from build123d import *

# Parameters (mm, degrees)
EXTRUDE_1_DEPTH          = 2.3
EXTRUDE_1_DEPTH_BACK     = 2.3
EXTRUDE_2_DEPTH          = 1.4
EXTRUDE_3_DEPTH          = 2
EXTRUDE_3_DEPTH_BACK     = 2
CUT_EXTRUDE_2_DEPTH      = 7.4
CUT_EXTRUDE_3_DEPTH      = 2
CUT_EXTRUDE_3_DEPTH_BACK = 2
FILLET_1_R               = 0.2
FILLET_2_R               = 0.1


with BuildPart() as part:
    # 草图1 → 凸台-拉伸1 (new, two sides: drawn at the far end of the back side and taken through both)
    with BuildSketch(Plane.XY.offset(-EXTRUDE_1_DEPTH_BACK)):
        Polygon((0, 0), (-14.8, 0), (-14.8, 1.3), (0, 1.3), (5.65072033, 1.3), (2.420449835, 19.619774331), (-0.822713256, 23.484825595), (-1.2165133, 23.484825595), (-1.2165133, 24.784825595), (-0.2165133, 24.784825595), (3.640212358, 20.188558937), (7.2, 0), align=None)
    extrude(amount=EXTRUDE_1_DEPTH + EXTRUDE_1_DEPTH_BACK)

    # 草图2 → 凸台-拉伸2 (add)
    with BuildSketch(Plane.XY.offset(2.3)):
        with BuildLine():
            Line((-14.8, 0), (7.2, 0))
            Line((7.2, 0), (3.640212358, 20.188558937))
            Line((3.640212358, 20.188558937), (-0.2165133, 24.784825595))
            Line((-0.2165133, 24.784825595), (-1.2165133, 24.784825595))
            ThreePointArc((-1.2165133, 24.784825595), (-2.266370135, 9.969308294), (-14.8, 2))
            Line((-14.8, 2), (-14.8, 0))
        make_face()
    extrude_2 = extrude(amount=EXTRUDE_2_DEPTH)

    # 镜向1: 凸台-拉伸2 across plane
    add(extrude_2.mirror(Plane.XY))

    # 草图4 → 凸台-拉伸3 (add, two sides: drawn at the far end of the back side and taken through both)
    with BuildSketch(Plane.XY.offset(-EXTRUDE_3_DEPTH_BACK)):
        with BuildLine():
            Line((-1.5, 0), (1.5, 0))
            Line((1.5, 0), (1.5, -0.677124344))
            ThreePointArc((1.5, -0.677124344), (1.780042303, -1.088161527), (1.95, -1.555590279))
            Line((1.95, -1.555590279), (1.95, -2.5))
            Line((1.95, -2.5), (-1.95, -2.5))
            Line((-1.95, -2.5), (-1.95, -1.555590279))
            ThreePointArc((-1.95, -1.555590279), (-1.780042303, -1.088161527), (-1.5, -0.677124344))
            Line((-1.5, -0.677124344), (-1.5, 0))
        make_face()
    extrude(amount=EXTRUDE_3_DEPTH + EXTRUDE_3_DEPTH_BACK)

    # 草图5 → 切除-拉伸2 (cut)
    with BuildSketch(Plane.XY.offset(3.7)):
        with BuildLine():
            Line((-1.2165133, 24.784825595), (-14.8, 2))
            ThreePointArc((-14.8, 2), (-2.266370135, 9.969308294), (-1.2165133, 24.784825595))
        make_face()
    extrude(amount=-CUT_EXTRUDE_2_DEPTH, mode=Mode.SUBTRACT)

    # 草图6 → 切除-拉伸3 (cut, two sides: drawn at the far end of the back side and taken through both)
    with BuildSketch(Plane(origin=(0, 0, 0), x_dir=(0, 0, -1), z_dir=(1, 0, 0)).offset(-CUT_EXTRUDE_3_DEPTH_BACK)):
        with BuildLine():
            Line((1.5, 0), (1.5, -0.677124344))
            ThreePointArc((1.5, -0.677124344), (1.780042303, -1.088161527), (1.95, -1.555590279))
            Line((1.95, -1.555590279), (1.95, -2.5))
            Line((1.95, -2.5), (2, -2.5))
            Line((2, -2.5), (2, 0))
            Line((2, 0), (1.5, 0))
        make_face()
        with BuildLine():
            Line((-1.95, -2.5), (-2, -2.5))
            Line((-2, -2.5), (-2, 0))
            Line((-2, 0), (-1.5, 0))
            Line((-1.5, 0), (-1.5, -0.677124344))
            ThreePointArc((-1.5, -0.677124344), (-1.780042303, -1.088161527), (-1.95, -1.555590279))
            Line((-1.95, -1.555590279), (-1.95, -2.5))
        make_face()
    extrude(amount=CUT_EXTRUDE_3_DEPTH + CUT_EXTRUDE_3_DEPTH_BACK, mode=Mode.SUBTRACT)

    # 圆角1
    fillet_1_edges = [part.edges().sort_by_distance(p)[0] for p in [
        (-14.8, 2, -3),
        (-14.8, 2, 3),
        (-14.8, 1, 3.7),
        (-14.8, 1, -3.7),
        (-0.7165133, 24.784825595, -3.7),
        (-0.7165133, 24.784825595, 3.7),
        (-0.2165133, 24.784825595, 0),
        (1.711849529, 22.486692266, -3.7),
        (1.711849529, 22.486692266, 3.7),
        (3.640212358, 20.188558937, 0),
        (5.420106179, 10.094279468, -3.7),
        (5.420106179, 10.094279468, 3.7),
        (7.2, 0, 0),
        (-3.8, 0, -3.7),
        (-3.8, 0, 3.7),
        (-14.8, 0, 0),
    ]]
    fillet(fillet_1_edges, radius=FILLET_1_R)

    # 圆角2
    fillet_2_edges = [part.edges().sort_by_distance(p)[0] for p in [
        (1.95, -2.5, 0),
        (-1.95, -2.5, 0),
        (0, -2.5, -1.95),
        (0, -2.5, 1.95),
    ]]
    fillet(fillet_2_edges, radius=FILLET_2_R)


solid = part.part
Input: part model. Units: mm. Frame: model coordinates. A direction names the side the tool comes from. Coordinates: 2 decimals unless noted, no trailing zeros. Write each loop counter-clockwise with the first axis right and the second up, starting at its lowest first coordinate (ties: lowest second). Pieces come first, ordered by that corner, then holes. Notation, with made-up numbers: M 34,42.5 L 84,42.5 A24 ccw 84,57.5 Z; hole C 6.25,9.5 d4. An arc over 180 degrees is marked long. Answer as a JSON object with one key per item and string values. Group by question number.
(1) Section B-B on x = -2.5. Output: boundary loops of the cut face in (y, z), plus the area to 3 significant figures.
(2) Ray query, line 1 along Z through (x, y) = (0.5, 13.75); line 2 along Y through (x, z) = (-7.5, 1.75); line 3 along Y through (x, z) = (2.25, 2.25). Return the intervals inside material, ascending. Write a range as [from, to].
(3) Set-up query: faces 4 (the face through (1.95, -2, 0)), 5 (the face through (-0.027, -1.082, -1.777)), 6 (the face through (-0.027, -1.082, 1.777)). Return all of +Z, -Z, +X, -X, +Y, -Y with unobstructed straight access to the full face (end or side cutting, diameter ignored); none if empty.
(4) Section C-C on z = -1. Output: boundary loops of the cut face in (x, y), plus the area to 3 significant figures.
(5) Mould query, pull axis Z, two halves, no side actions, for faces 1 (the face through (-1.78, -1.09, -0.03)), 2 (the face through (0, -2, 1.95)), 3 (the face through (0, 7, 2.3)). Classes: pulls with the +Z half, pulls with the -Z half, needs draft (parallel to the pull), parting line crosses it, or undercut.
(6) Section D-D on x = -10.5. Output: boundary loops of the cut face in (y, z).
(7) Section A-A on z = -2.75. Output: boundary loops of the cut face in (x, y).
(8) Contact query for flat-ended pins moving along their axis: P1, Ø0.7, axis at x = 0, y = 0, coming from the -Z side; P2, Ø0.7, axis at y = -0.5, z = 0, coming from the +X side; P3, Ø1, axis at y = 8.5, z = -2.5, coming from the -X side; P4, Ø0.7, axis at y = -2, z = 0.5, coming from the -X side. Output: stop coordinate, or through.
Result set:
{
 "1": {"outline": "M 0,-3.5 A0.2 ccw 0.2,-3.7 L 9.59,-3.7 L 9.59,-2.3 L 1.3,-2.3 L 1.3,2.3 L 9.59,2.3 L 9.59,3.7 L 0.2,3.7 A0.2 ccw 0,3.5 Z", "area": "32.8 mm2"},
 "2": {"line 1": "z = [-3.7, -2.3], [2.3, 3.7]", "line 2": "y = [0, 1.3]", "line 3": "y = [0, 1.3], [19.82, 21.85]"},
 "3": {"face 4": "+Z, -Z, +X, -Y", "face 5": "-Z, +X, -X", "face 6": "+Z, +X, -X"},
 "4": {"outline": "M -14.8,0.2 A0.2 ccw -14.6,0 L -1.5,0 L -1.5,-0.68 A2 ccw -1.95,-1.56 L -1.95,-2.4 A0.1 ccw -1.85,-2.5 L 1.85,-2.5 A0.1 ccw 1.95,-2.4 L 1.95,-1.56 A2 ccw 1.5,-0.68 L 1.5,0 L 6.96,0 A0.2 ccw 7.16,0.23 L 3.65,20.14 A0.2 ccw 3.61,20.23 L -0.16,24.71 A0.2 ccw -0.31,24.78 L -1.22,24.78 A16.5 cw -0.68,23.32 L 2.42,19.62 L 5.65,1.3 L -14.8,1.3 Z", "area": "69.6 mm2"},
 "5": {"face 1": "needs draft", "face 2": "pulls with the +Z half", "face 3": "undercut"},
 "6": {"outline": "M 0,-3.5 A0.2 ccw 0.2,-3.7 L 3.02,-3.7 L 3.02,-2.3 L 1.3,-2.3 L 1.3,2.3 L 3.02,2.3 L 3.02,3.7 L 0.2,3.7 A0.2 ccw 0,3.5 Z"},
 "7": {"outline": "M -14.8,0.2 A0.2 ccw -14.6,0 L 6.96,0 A0.2 ccw 7.16,0.23 L 3.65,20.14 A0.2 ccw 3.61,20.23 L -0.16,24.71 A0.2 ccw -0.31,24.78 L -1.22,24.78 A16.5 cw -14.62,2.02 A0.2 ccw -14.8,1.82 Z"},
 "8": {"P1": "stops at z = -3.7", "P2": "stops at x = 1.64", "P3": "stops at x = -3.64", "P4": "stops at x = -1.95"}
}
